from build123d import *

# Parameters (mm, degrees)
SKETCH1_R           = 4.2
SKETCH1_R_2         = 2.7
SKETCH1_R_3         = 2.2
SKETCH1_R_4         = 26.2
BOSS_EXTRUDE1_DEPTH = 10.3
SKETCH2_R           = 5.2
CUT_EXTRUDE2_DEPTH  = 5.2
CHAMFER1_SIZE       = 0.4


with BuildPart() as part:
    # Sketch1 → Boss-Extrude1 (new body)
    with BuildSketch(Plane(origin=(0, 0, 0), x_dir=(1, 0, 0), z_dir=(0, 1, 0))):
        with BuildLine():
            Line((161.746435314, 45.617999491), (13.995662136, 73.682572169))
            ThreePointArc((13.995662136, 73.682572169), (-75, 0), (13.995662136, -73.682572169))
            Line((13.995662136, -73.682572169), (161.746435314, -45.617999491))
            ThreePointArc((161.746435314, -45.617999491), (164.081050248, -44.239169867), (165, -41.688262309))
            Line((165, -41.688262309), (165, 0))
            Line((165, 0), (165, 41.688262309))
            ThreePointArc((165, 41.688262309), (164.081050248, 44.239169867), (161.746435314, 45.617999491))
        make_face()
        with Locations(Location((-40, -50, 0), (0, 0, 90))):
            Circle(SKETCH1_R, mode=Mode.SUBTRACT)
        with Locations(Location((0, -50.35, 0), (0, 0, 90))):
            Circle(SKETCH1_R_2, mode=Mode.SUBTRACT)
        with Locations(Location((-43.604379081, -25.175, 0), (0, 0, 90))):
            Circle(SKETCH1_R_2, mode=Mode.SUBTRACT)
        with Locations(Location((43.604379081, -25.175, 0), (0, 0, 90))):
            Circle(SKETCH1_R_2, mode=Mode.SUBTRACT)
        with Locations(Location((60, -50, 0), (0, 0, 90))):
            Circle(SKETCH1_R, mode=Mode.SUBTRACT)
        with Locations(Location((104.75, -25.5, 0), (0, 0, 90))):
            Circle(SKETCH1_R_3, mode=Mode.SUBTRACT)
        with Locations(Location((129.25, -25.5, 0), (0, 0, 90))):
            Circle(SKETCH1_R_3, mode=Mode.SUBTRACT)
        with Locations(Location((-43.604379081, 25.175, 0), (0, 0, 90))):
            Circle(SKETCH1_R_2, mode=Mode.SUBTRACT)
        with Locations(Location((0, 0, 0), (0, 0, 90))):
            Circle(SKETCH1_R_4, mode=Mode.SUBTRACT)
        with Locations(Location((43.604379081, 25.175, 0), (0, 0, 90))):
            Circle(SKETCH1_R_2, mode=Mode.SUBTRACT)
        with Locations(Location((-40, 50, 0), (0, 0, 90))):
            Circle(SKETCH1_R, mode=Mode.SUBTRACT)
        with Locations(Location((0, 50.35, 0), (0, 0, 90))):
            Circle(SKETCH1_R_2, mode=Mode.SUBTRACT)
        with Locations(Location((104.75, 25.5, 0), (0, 0, 90))):
            Circle(SKETCH1_R_3, mode=Mode.SUBTRACT)
        with BuildLine():
            ThreePointArc((122, 18.5), (140.5, 0), (122, -18.5))
            Line((122, -18.5), (112, -18.5))
            ThreePointArc((112, -18.5), (93.5, 0), (112, 18.5))
            Line((112, 18.5), (122, 18.5))
        make_face(mode=Mode.SUBTRACT)
        with Locations(Location((129.25, 25.5, 0), (0, 0, 90))):
            Circle(SKETCH1_R_3, mode=Mode.SUBTRACT)
        with Locations(Location((60, 50, 0), (0, 0, 90))):
            Circle(SKETCH1_R, mode=Mode.SUBTRACT)
    extrude(amount=BOSS_EXTRUDE1_DEPTH)

    # Sketch2 → Cut-Extrude2 (cut)
    with BuildSketch(Plane.XZ):
        with Locations(Location((43.604379081, -25.175, 0), (0, 0, 270))):
            Circle(SKETCH2_R)
        with Locations(Location((0, -50.35, 0), (0, 0, 270))):
            Circle(SKETCH2_R)
        with Locations(Location((-43.604379081, -25.175, 0), (0, 0, 270))):
            Circle(SKETCH2_R)
        with Locations(Location((-43.604379081, 25.175, 0), (0, 0, 270))):
            Circle(SKETCH2_R)
        with Locations(Location((0, 50.35, 0), (0, 0, 270))):
            Circle(SKETCH2_R)
        with Locations(Location((43.604379081, 25.175, 0), (0, 0, 270))):
            Circle(SKETCH2_R)
        with Locations(Location((104.75, -25.5, 0), (0, 0, 270))):
            Circle(SKETCH2_R)
        with Locations(Location((129.25, -25.5, 0), (0, 0, 270))):
            Circle(SKETCH2_R)
        with Locations(Location((129.25, 25.5, 0), (0, 0, 270))):
            Circle(SKETCH2_R)
        with Locations(Location((104.75, 25.5, 0), (0, 0, 270))):
            Circle(SKETCH2_R)
    extrude(amount=-CUT_EXTRUDE2_DEPTH, mode=Mode.SUBTRACT)

    # Chamfer1
    chamfer1_edges = [part.edges().sort_by_distance(p)[0] for p in [
        (-43.604379081, 5.2, -22.475),
        (164.081050248, 10.3, 44.239169867),
        (-43.604379081, 0, -19.975),
        (0, 5.2, -47.65),
        (0, 0, -45.15),
        (165, 10.3, 0),
        (104.75, 0, -20.3),
        (104.75, 5.2, -23.3),
        (104.75, 5.2, 27.7),
        (104.75, 0, 30.7),
        (164.081050248, 10.3, -44.239169867),
        (43.604379081, 5.2, -22.475),
        (43.604379081, 0, -19.975),
        (87.871048725, 10.3, -59.65028583),
        (-75, 10.3, 0),
        (0, 10.3, 26.2),
        (-43.604379081, 10.3, -22.475),
        (-75, 0, 0),
        (87.871048725, 0, -59.65028583),
        (164.081050248, 0, -44.239169867),
        (60, 10.3, -45.8),
        (165, 0, 0),
        (164.081050248, 0, 44.239169867),
        (87.871048725, 0, 59.65028583),
        (-40, 0, -45.8),
        (117, 0, 18.5),
        (140.5, 0, 0),
        (0, 10.3, 53.05),
        (117, 0, -18.5),
        (93.5, 0, 0),
        (-40, 0, 54.2),
        (60, 10.3, 54.2),
        (60, 0, 54.2),
        (60, 0, -45.8),
        (0, 0, 26.2),
        (43.604379081, 10.3, 27.875),
        (-40, 10.3, 54.2),
        (43.604379081, 10.3, -22.475),
        (0, 10.3, -47.65),
        (129.25, 10.3, -23.3),
        (129.25, 10.3, 27.7),
        (104.75, 10.3, 27.7),
        (93.5, 10.3, 0),
        (117, 10.3, -18.5),
        (140.5, 10.3, 0),
        (117, 10.3, 18.5),
        (104.75, 10.3, -23.3),
        (129.25, 5.2, 27.7),
        (129.25, 0, 30.7),
        (-43.604379081, 10.3, 27.875),
        (129.25, 0, -20.3),
        (129.25, 5.2, -23.3),
        (43.604379081, 5.2, 27.875),
        (43.604379081, 0, 30.375),
        (-40, 10.3, -45.8),
        (0, 5.2, 53.05),
        (0, 0, 55.55),
        (87.871048725, 10.3, 59.65028583),
        (-43.604379081, 5.2, 27.875),
        (-43.604379081, 0, 30.375),
    ]]
    chamfer(chamfer1_edges, length=CHAMFER1_SIZE)


solid = part.part
Model file for the job. Use its own axes, mm. A direction names the side the tool comes from. Coordinates: 2 decimals unless noted, no trailing zeros. Write each loop counter-clockwise with the first axis right and the second up, starting at its lowest first coordinate (ties: lowest second). Pieces come first, ordered by that corner, then holes. Notation, with made-up numbers: (11.25, 17) -> (57.25, 17) arc R19 cw to (57.25, 37) -> close; hole circle Ø3 at (62.5, 67). An arc over 180 degrees is marked (long way). One line per item, written item: value. Start each with the question number.
1) Which spindle directions (+Z, -Z, +X, -X, +Y, -Y) get a long thin tool onto all of the face, cutting with end or side? Do faces 1 (the face through (-46.28, 7.72, -24.82)), 2 (the face through (132, 5.2, 24)), 3 (the face through (140.604, 10.008, -0.409)). Say none if no direction does.
2) Probe probe 1 along X at (y, z) = (7, 1); probe 2 along X at (y, z) = (7.25, -2.5); probe 3 along X at (y, z) = (6, -24). List the from-to ranges inside material, lowest first.
3) Flat gauge pins, fed straight in: pin 1 Ø13.5 at (x, z) = (129.25, 25.5) entering from +Y; pin 2 Ø6 at (x, z) = (-43.6, 25.18) entering from +Y; pin 3 Ø5 at (x, y) = (117.5, 3.5) entering from -Z; pin 4 Ø4.5 at (x, z) = (43.6, -25.18) entering from +Y. Where does each tip first touch, or does it go through?
4) Slice it at B-B on x = 88. Write the cut outline in (y, z), then the cut area to 3 significant figures.
5) Slice it at A-A on y = 3. Count the separate pieces of the cut face and the enclosed holes in it, then the cut area to 3 significant figures.
6) Pull direction Z, two halves, no side cores. Call faces 4 (the face through (-0.119, 7.72, -47.653)), 5 (the face through (86.8, 10.1, 59.65)): +Z half, -Z half, draft (parallel to the pull), parting line (faces both ways), or undercut.
Answers follow:
1. face 1: +Y, -Y
1. face 2: -Y
1. face 3: +Y
2. probe 1: -74.99 to -26.18, 26.18 to 93.53, 140.47 to 165
2. probe 2: -74.96 to -26.08, 26.08 to 93.67, 140.33 to 165
2. probe 3: -71.06 to -46.04, -41.17 to -10.51, 10.51 to 41.17, 46.04 to 103.14, 106.36 to 127.64, 130.86 to 165
3. pin 1: y = 10.3
3. pin 2: y = 10.21
3. pin 3: z = -54.5
3. pin 4: through
4. outline: (0, -59.22) -> (0.4, -59.63) -> (9.9, -59.63) -> (10.3, -59.22) -> (10.3, 59.22) -> (9.9, 59.63) -> (0.4, 59.63) -> (0, 59.22) -> close
4. area: 1,230 mm2
5. separate pieces: 1
5. enclosed holes: 16
5. area: 24,200 mm2
6. face 4: undercut
6. face 5: +Z half
